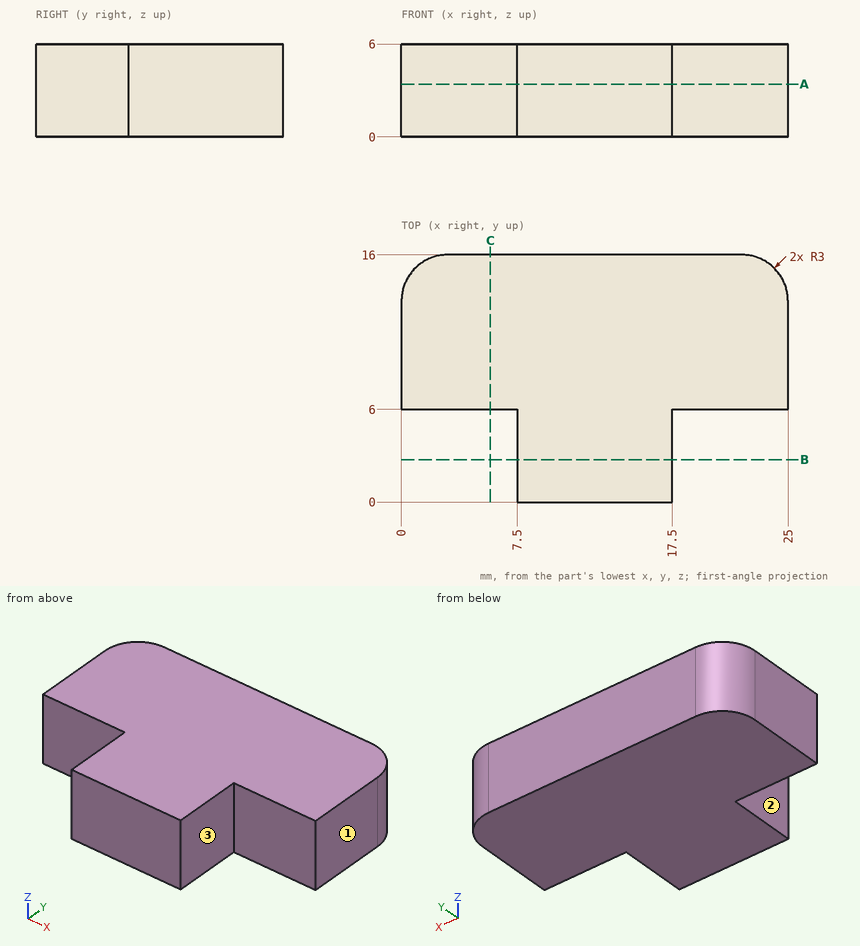
For this review, use the dimensioned drawing (mm, ordinates from the lowest corner) and the shaded views. A direction names the side the tool comes from. Coordinates: 2 decimals unless noted, no trailing zeros. Loops run counter-clockwise (first coordinate to the right, second up) from the corner with the lowest first, then second, coordinate; pieces in that order, holes last.
1. For line 1 (Y direction, x = 18, z = 1); line 2 (X direction, y = 3.5, z = 2.75); line 3 (X direction, y = 13.75, z = 3.9), list the stretches that pass through material, from the lowest coordinate up.
2. Insertion check: P1, Ø3, axis at x = 3.5, z = 3, coming from the -Y side. The pin has a flat end and moves straight along its axis. Give the tip position at first contact, or say it passes through.
3. Add section B-B, the plane y = 2.75. Give the boundary of the cut face in (x, z), then the cut area to 3 significant figures.
4. Add section A-A, the plane z = 3.4. Give the boundary of the cut face in (x, y), then the cut area to 3 significant figures.
5. For the marked faces 1, 2 and 3, list the 3-axis set-ups (+Z, -Z, +X, -X, +Y, -Y) from which the entire face can be reached by the end or side of a thin tool; tool diameter is ignored.
6. Add section C-C, the plane x = 5.75. Give the boundary of the cut face in (y, z).
Result:
1. line 1: y = 6 to 16
1. line 2: x = 7.5 to 17.5
1. line 3: x = 0.1 to 24.9
2. P1: stops at y = 6
3. outline: (7.5, 0) - (17.5, 0) - (17.5, 6) - (7.5, 6) - close
3. area: 60.0 mm2
4. outline: (0, 6) - (7.5, 6) - (7.5, 0) - (17.5, 0) - (17.5, 6) - (25, 6) - (25, 13) arc R3 ccw to (22, 16) - (3, 16) arc R3 ccw to (0, 13) - close
4. area: 306 mm2
5. face 1: +Z, -Z, +X, +Y, -Y
5. face 2: +Z, -Z, -X, -Y
5. face 3: +Z, -Z, +X, -Y
6. outline: (6, 0) - (16, 0) - (16, 6) - (6, 6) - close
